```python
from build123d import *

# Parameters (mm, degrees)
SKETCH1_R           = 11
BOSS_EXTRUDE2_DEPTH = 5.65
SKETCH3_R           = 2.8
SKETCH3_R_2         = 1.5
CUT_EXTRUDE2_DEPTH  = 12
CUT_EXTRUDE3_START  = -4
SKETCH4_R           = 11
SKETCH4_R_2         = 4.5
CUT_EXTRUDE3_DEPTH  = 4
SKETCH5_W           = 9
SKETCH5_H           = 0.6
CUT_EXTRUDE4_DEPTH  = 18
SKETCH6_R           = 2.8
SKETCH6_R_2         = 1.5
BOSS_EXTRUDE4_DEPTH = 2.3
SKETCH7_R           = 11
SKETCH7_R_2         = 2.8
SKETCH7_R_3         = 1.5
BOSS_EXTRUDE5_DEPTH = 0.7


with BuildPart() as part:
    # Sketch1 → Boss-Extrude2 (new body)
    with BuildSketch(Plane(origin=(0, 0, 0), x_dir=(1, 0, 0), z_dir=(0, 1, 0))):
        with Locations(Location((0, 0, 0), (0, 0, 270))):
            Circle(SKETCH1_R)
    extrude(amount=BOSS_EXTRUDE2_DEPTH)

    # Sketch3 → Cut-Extrude2 (cut)
    with BuildSketch(Plane(origin=(0, 5.65, 0), x_dir=(1, 0, 0), z_dir=(0, 1, 0))):
        with Locations(Location((0, 0, 0), (0, 0, 270))):
            Circle(SKETCH3_R)
        with Locations(Location((-6.9, 0, 0), (0, 0, 270))):
            Circle(SKETCH3_R_2)
        with Locations(Location((0, 6.9, 0), (0, 0, 270))):
            Circle(SKETCH3_R_2)
        with Locations(Location((6.9, 0, 0), (0, 0, 270))):
            Circle(SKETCH3_R_2)
        with Locations(Location((0, -6.9, 0), (0, 0, 270))):
            Circle(SKETCH3_R_2)
    extrude(amount=-CUT_EXTRUDE2_DEPTH, mode=Mode.SUBTRACT)

    # Sketch4 → Cut-Extrude3 (cut)
    with BuildSketch(Plane(origin=(0, 5.65, 0), x_dir=(1, 0, 0), z_dir=(0, 1, 0)).offset(CUT_EXTRUDE3_START)):
        with Locations(Location((0, 0, 0), (0, 0, 270))):
            Circle(SKETCH4_R)
        with Locations(Location((0, 0, 0), (0, 0, 270))):
            Circle(SKETCH4_R_2, mode=Mode.SUBTRACT)
    extrude(amount=CUT_EXTRUDE3_DEPTH, mode=Mode.SUBTRACT)

    # Sketch5 → Cut-Extrude4 (cut)
    with BuildSketch(Plane(origin=(10, 0, 0), x_dir=(0, 0, -1), z_dir=(1, 0, 0))):
        with Locations((0, 5.35)):
            Rectangle(SKETCH5_W, SKETCH5_H)
    extrude(amount=-CUT_EXTRUDE4_DEPTH, mode=Mode.SUBTRACT)

    # Sketch6 → Boss-Extrude4 (add)
    with BuildSketch(Plane(origin=(0, 1.65, 0), x_dir=(1, 0, 0), z_dir=(0, 1, 0))):
        with Locations(Location((0, 0, 0), (0, 0, 270))):
            Circle(SKETCH6_R)
        with Locations(Location((0, 0, 0), (0, 0, 270))):
            Circle(SKETCH6_R_2, mode=Mode.SUBTRACT)
    extrude(amount=-BOSS_EXTRUDE4_DEPTH)

    # Sketch7 → Boss-Extrude5 (add)
    with BuildSketch(Plane.XZ):
        with Locations(Location((0, 0, 0), (0, 0, 270))):
            Circle(SKETCH7_R)
        with Locations(Location((0, 0, 0), (0, 0, 90))):
            Circle(SKETCH7_R_2, mode=Mode.SUBTRACT)
        with Locations(Location((0, 6.9, 0), (0, 0, 90))):
            Circle(SKETCH7_R_3, mode=Mode.SUBTRACT)
        with Locations(Location((6.9, 0, 0), (0, 0, 90))):
            Circle(SKETCH7_R_3, mode=Mode.SUBTRACT)
        with Locations(Location((0, -6.9, 0), (0, 0, 90))):
            Circle(SKETCH7_R_3, mode=Mode.SUBTRACT)
        with Locations(Location((-6.9, 0, 0), (0, 0, 90))):
            Circle(SKETCH7_R_3, mode=Mode.SUBTRACT)
    extrude(amount=BOSS_EXTRUDE5_DEPTH)


solid = part.part
```
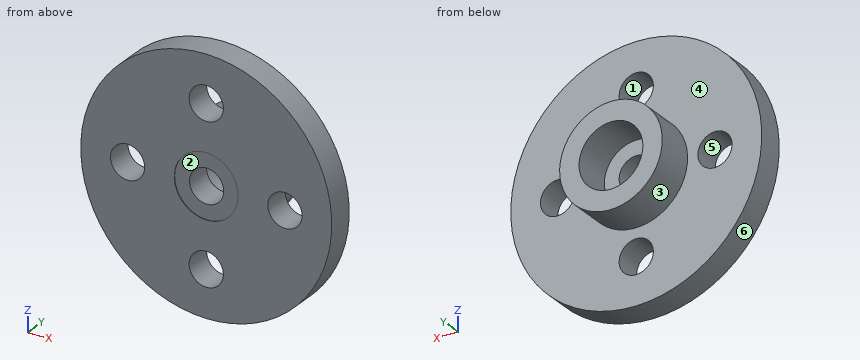
The listing builds one solid part. Answer for the finished solid, in the listing's coordinates (mm). Face numbers are marked on the shaded views. A direction names the side the tool comes from. Round coordinates to 2 decimals unless told otherwise and drop trailing zeros. Write each loop counter-clockwise with the first axis right and the second up, starting at its lowest first coordinate (ties: lowest second). Pieces come first, ordered by that corner, then holes. Notation, with made-up numbers: (11, 3.25) -> (55, 3.25) arc R26 cw to (55, 24.25) -> close; hole circle Ø4 at (77, 67.5). An arc over 180 degrees is marked (long way). Write item = value, one per line.
1) Section D-D on z = -6.9 is taken. Write down the section's boundary in (x, y).
Check values:
outline = (-8.57, -0.7) -> (-1.5, -0.7) -> (-1.5, 1.65) -> (-8.57, 1.65) -> close; (1.5, -0.7) -> (8.57, -0.7) -> (8.57, 1.65) -> (1.5, 1.65) -> close
2) Given pin 1 (2.5 mm diameter, centred on x = 0, z = -6.9, fed in from -Y); pin 2 (3 mm diameter, centred on x = -0.5, z = 0, fed in from +Y); pin 3 (5 mm diameter, centred on x = 0, z = 0, fed in from -Y); pin 4 (1 mm diameter, centred on y = 4, z = -3.5, fed in from +X), each flat-ended and moving along its own axis, determine where each tip first touches the part or whether it passes through.
Check values:
pin_1 = through
pin_2 = 1.65
pin_3 = -0.65
pin_4 = 3.35
3) Section C-C on y = 0.5 is taken. Write down the section's boundary in (x, z).
Check values:
outline = circle Ø22 at (0, 0); hole circle Ø3 at (-6.9, 0); hole circle Ø3 at (0, -6.9); hole circle Ø3 at (0, 0); hole circle Ø3 at (0, 6.9); hole circle Ø3 at (6.9, 0)
4) Which of the six approach directions +Z, -Z, +X, -X, +Y, -Y give full straight-line access (tool end or side, diameter ignored) to the marked faces 1, 2 and 3?
Check values:
face_1 = +Y, -Y
face_2 = -Y
face_3 = +Y
5) Section A-A on z = 0 is taken. Write down the section's boundary in (x, y), plus the area to 3 significant figures.
Check values:
outline = (-11, -0.7) -> (-8.4, -0.7) -> (-8.4, 1.65) -> (-11, 1.65) -> close; (-5.4, -0.7) -> (-2.8, -0.7) -> (-2.8, -0.65) -> (-1.5, -0.65) -> (-1.5, 1.65) -> (-2.8, 1.65) -> (-2.8, 5.05) -> (-4.5, 5.05) -> (-4.5, 1.65) -> (-5.4, 1.65) -> close; (1.5, -0.65) -> (2.8, -0.65) -> (2.8, -0.7) -> (5.4, -0.7) -> (5.4, 1.65) -> (4.5, 1.65) -> (4.5, 5.05) -> (2.8, 5.05) -> (2.8, 1.65) -> (1.5, 1.65) -> close; (8.4, -0.7) -> (11, -0.7) -> (11, 1.65) -> (8.4, 1.65) -> close
area = 42.0 mm²
6) Section B-B on x = 0 is taken. Write down the section's boundary in (y, z).
Check values:
outline = (-0.7, -11) -> (1.65, -11) -> (1.65, -8.4) -> (-0.7, -8.4) -> close; (-0.7, -5.4) -> (1.65, -5.4) -> (1.65, -4.5) -> (5.05, -4.5) -> (5.05, -2.8) -> (1.65, -2.8) -> (1.65, -1.5) -> (-0.65, -1.5) -> (-0.65, -2.8) -> (-0.7, -2.8) -> close; (-0.7, 2.8) -> (-0.65, 2.8) -> (-0.65, 1.5) -> (1.65, 1.5) -> (1.65, 2.8) -> (5.05, 2.8) -> (5.05, 4.5) -> (1.65, 4.5) -> (1.65, 5.4) -> (-0.7, 5.4) -> close; (-0.7, 8.4) -> (1.65, 8.4) -> (1.65, 11) -> (-0.7, 11) -> close
7) Straight lines are drawn through the part: line 1 along X through (y, z) = (3, 0); line 2 along X through (y, z) = (1.2, 1.25); line 3 along Y through (x, z) = (3.75, 9.25). For each, find the intervals that lie inside material, in ascending order. Write a range as [from, to].
Check values:
line_1 = [-4.5, -2.8], [2.8, 4.5]
line_2 = [-10.93, -7.73], [-6.07, -0.83], [0.83, 6.07], [7.73, 10.93]
line_3 = [-0.7, 1.65]
8) For a pull along Z with two mould halves and no side action, classify the marked faces 4, 5 and 6 as released by +Z, released by -Z, zero draft, split by the parting line, or undercut.
Check values:
face_4 = zero draft
face_5 = undercut
face_6 = split by the parting line
